from build123d import *

# Parameters (mm, degrees)
SKETCH_1_R      = 1.5
EXTRUDE_1_DEPTH = 4


with BuildPart() as part:
    # 草图1 → 凸台-拉伸1 (new body)
    with BuildSketch(Plane.XY):
        Polygon((-7, 7), (65.12, 7), (65.12, -8), (43.12, -8), (43.12, -26), (15, -26), (15, -8), (-7, -8), align=None)
        Circle(SKETCH_1_R, mode=Mode.SUBTRACT)
        with Locations((58.12, 0)):
            Circle(SKETCH_1_R, mode=Mode.SUBTRACT)
    extrude(amount=EXTRUDE_1_DEPTH)


solid = part.part
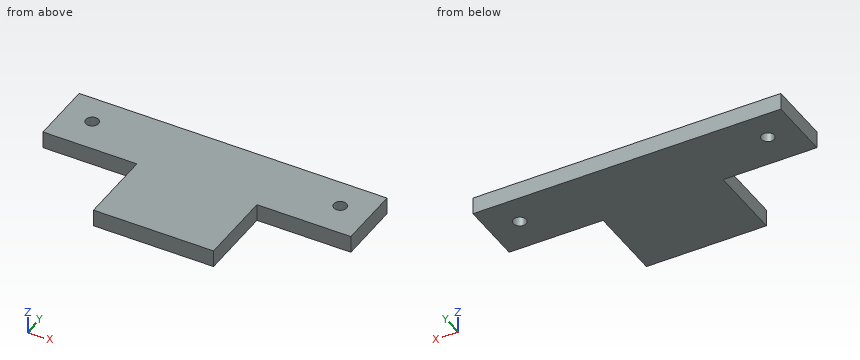
CAD build for the part. Positions are in the model's coordinates, mm. Round coordinates to 2 decimals unless told otherwise and drop trailing zeros. Order: outer loops, then holes, each group sorted by start corner. A loop starts at its lowest first (then second) coordinate and runs counter-clockwise, first axis right, second up. Notation, with made-up numbers: (52.25, 29.5) - (102.25, 29.5) arc R27 ccw to (102.25, 50.5) - close; hole circle Ø2 at (23, 5.5). An arc over 180 degrees is marked (long way). Return JSON: item names as keys, results as strings.
(1) Cut at D-D (x = 3). Give the cut face in (y, z), then the cut area to 3 significant figures.
Answer key:
{"outline": "(-8, 0) - (7, 0) - (7, 4) - (-8, 4) - close", "area": "60.0 mm^2"}
(2) Pin check, flat tips, straight feed: pin 1 Ø2 at (x, z) = (9.5, 2) entering from -Y; pin 2 Ø1.2 at (y, z) = (-15.5, 2) entering from +X; pin 3 Ø1.2 at (y, z) = (-19, 2) entering from -X. Stop position of each tip, or through.
Answer key:
{"pin 1": "stops at y = -8", "pin 2": "stops at x = 43.12", "pin 3": "stops at x = 15"}
(3) Cut at C-C (x = 58.12). Give the cut face in (y, z).
Answer key:
{"outline": "(-8, 0) - (-1.5, 0) - (-1.5, 4) - (-8, 4) - close; (1.5, 0) - (7, 0) - (7, 4) - (1.5, 4) - close"}
(4) Cut at B-B (z = 2.05). Give the cut face in (x, y), then the cut area to 3 significant figures.
Answer key:
{"outline": "(-7, -8) - (15, -8) - (15, -26) - (43.12, -26) - (43.12, -8) - (65.12, -8) - (65.12, 7) - (-7, 7) - close; hole circle Ø3 at (0, 0); hole circle Ø3 at (58.12, 0)", "area": "1,570 mm^2"}
(5) Cut at A-A (y = 0). Give the cut face in (x, z), then the cut area to 3 significant figures.
Answer key:
{"outline": "(-7, 0) - (-1.5, 0) - (-1.5, 4) - (-7, 4) - close; (1.5, 0) - (56.62, 0) - (56.62, 4) - (1.5, 4) - close; (59.62, 0) - (65.12, 0) - (65.12, 4) - (59.62, 4) - close", "area": "264 mm^2"}
(6) Wall check: probe 1 along Y at (x, z) = (58.12, 2.6); probe 2 along Y at (x, z) = (-3, 1.95); probe 3 along X at (y, z) = (-11, 2.25). Give the ranges that are in metal, low to high. Write a range as from..to.
Answer key:
{"probe 1": "y = -8..-1.5, 1.5..7", "probe 2": "y = -8..7", "probe 3": "x = 15..43.12"}
